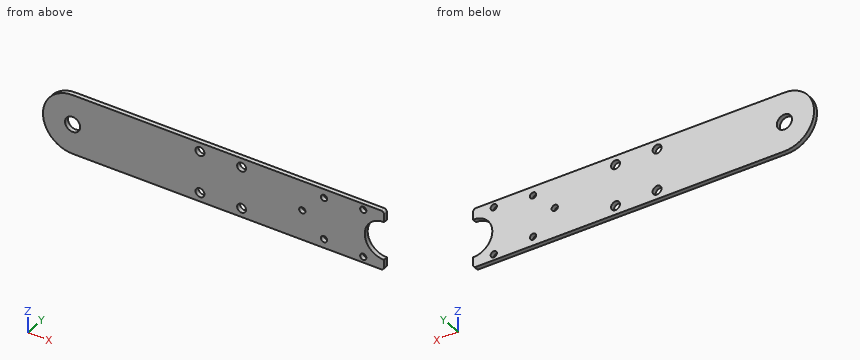
Autodesk Inventor part; units mm, degrees
ref_plane "YZ Plane" through (0, 0, 0) normal (1, 0, 0) x (0, 1, 0)
ref_plane "XZ Plane" through (0, 0, 0) normal (0, 1, 0) x (-1, 0, 0)
ref_plane "XY Plane" through (0, 0, 0) normal (0, 0, 1) x (1, 0, 0)
sketch "Sketch1" plane through (0, 0, 0) normal (0, 1, 0) x (-1, 0, 0)
  line L0 (-37.7289, 0) -> (-37.7289, -20)
  line L1 (-0.4496, -20) -> (-0.4496, 0)
  circle A0 centre (-64.5686, -18) radius 1.05
  circle A1 centre (-51.3486, -17) radius 1.05
  circle A2 centre (-44.0486, -10) radius 1.05
  circle A3 centre (-51.3486, -3) radius 1.05
  circle A4 centre (-64.5686, -2) radius 1.05
  circle A5 centre (-23.5893, -3) radius 1.5
  circle A6 centre (-9.5893, -3) radius 1.5
  circle A7 centre (-23.5893, -17) radius 1.5
  circle A8 centre (-9.5893, -17) radius 1.5
  circle A9 centre (33.29, -10) radius 2.55
  arc A10 (-70.5686, 0) -> (-71.5686, -1) centre (-70.5686, -1) ccw
  line L2 (-71.5686, -1) -> (-71.5686, -3.6008)
  arc A11 (-71.5686, -19) -> (-70.5686, -20) centre (-70.5686, -19) ccw
  line L3 (-71.5686, -16.3992) -> (-71.5686, -19)
  arc A12 (-71.5686, -16.3992) -> (-71.5686, -3.6008) centre (-71.4686, -10) ccw
  line L4 (-70.5686, 0) -> (33.29, 0)
  line L5 (33.29, -20) -> (-70.5686, -20)
  arc A13 (33.29, -20) -> (33.29, 0) centre (33.29, -10) ccw
  line L6 (-38.1786, -20) -> (-38.1786, 0)
  line L7 (-37.2793, 0) -> (-37.2793, -20)
  line L8 (-0.8993, -20) -> (-0.8993, 0)
  line L9 (0, 0) -> (0, -20)
  point P0 (0, 0)
extrude "Extrusion1" add sketch "Sketch1" against normal blind 1.5
properties part number "CAM_axis_3_bottom_frame"
Input: part model. Units: mm. Frame: model coordinates. Round coordinates to 2 decimals unless told otherwise and drop trailing zeros. Write each loop counter-clockwise with the first axis right and the second up, starting at its lowest first coordinate (ties: lowest second). Pieces come first, ordered by that corner, then holes. Notation, with made-up numbers: M 59,21 L 63,21 A19 cw 63,57 Z; hole C 46,25.5 d11. An arc over 180 degrees is marked long. Write each question's results on one line, items separated by ' | '.
Q1. Line query: line 1 along X through (y, z) = (-1.25, -9.5); line 2 along X through (y, z) = (-0.7, -2.5); line 3 along X through (y, z) = (-0.7, -18.25). Output: solid intervals per line, ascending.
Results:
line 1: x = -43.28 to -35.79, -30.79 to 43.13, 44.97 to 65.09 | line 2: x = -39.9 to 8.18, 11 to 22.18, 25 to 50.43, 52.27 to 63.65, 65.49 to 71.57 | line 3: x = -38.94 to 8.76, 10.42 to 22.76, 24.42 to 63.55, 65.59 to 71.57
Q2. Section query A-A (z = -10). Return loops of the section in (x, y).
Results:
outline: M -43.29,-1.5 L -35.84,-1.5 L -35.84,0 L -43.29,0 Z; M -30.74,-1.5 L 43,-1.5 L 43,0 L -30.74,0 Z; M 45.1,-1.5 L 65.07,-1.5 L 65.07,0 L 45.1,0 Z
Q3. Section query B-B (y = -0.85). State how many separate pieces and enclosed holes the cut face has, and give its area (3 significant figures).
Results:
separate pieces: 1 | enclosed holes: 10 | area: 2,120 mm^2
